Part model, mm, in its own coordinate system. A direction names the side the tool comes from. Give positions to 0.01 mm unless a question says otherwise; leave off trailing zeros. Write each loop counter-clockwise with the first axis right and the second up, starting at its lowest first coordinate (ties: lowest second). Pieces come first, ordered by that corner, then holes. Notation, with made-up numbers: M 8.5,-3.75 L 13.5,-3.75 A21 ccw 13.5,20.25 Z; hole C 28,-6.5 d11. An arc over 180 degrees is marked long. Answer as CSV lines item,"result". Start each with the question number.
1) Mould opens along X. For faces 1 (the flat face through (0, -17.5, -2)), 2 (the flat face through (-14.5, 0, -2)), 3 (the flat face through (17.5, 0, -2)) say: pulls with the +X half, pulls with the -X half, needs draft (parallel to the pull), parting line crosses it, or undercut.
2) Pin check, flat tip, straight feed: pin 1 Ø5 at (y, z) = (0, 56) entering from +X. Stop position of the tip, or through.
3) Slice it at A-A, the plane y = -12. Give the cut face in (x, z), plus the area to 3 significant figures.
4) Slice it at B-B, the plane z = 56. Give the cut face in (x, y), plus the area to 3 significant figures.
5) Slice it at D-D, the plane y = 0. Give the cut face in (x, z), plus the area to 3 significant figures.
6) Tool access for faces 4 (the flat face through (0, 14.5, -2)), 5 (the flat face through (-17.5, 0, -2)): list every direction of +Z, -Z, +X, -X, +Y, -Y with a clear straight run to the whole face (end or side of a thin tool).
7) Wall check: line 1 along Y through (x, z) = (15.8, 56); line 2 along X through (y, z) = (-11, -101.5). Give the ranges that are in metal, low to high. Write a range as from..to.
```python
from build123d import *

# Parameters (mm, degrees)
EXTRUDE_THIN1_DEPTH      = 140
EXTRUDE_THIN1_DEPTH_BACK = 140
SKETCH1_W                = 35
SKETCH1_H                = 35
SKETCH1_W_2              = 29
SKETCH1_H_2              = 29
FILLET1_R                = 2
SKETCH2_R                = 4
CUT_EXTRUDE1_DEPTH       = 40


with BuildPart() as part:
    # Sketch1 → Extrude-Thin1 (new, two sides: drawn at the far end of the back side and taken through both)
    with BuildSketch(Plane.XY.offset(-EXTRUDE_THIN1_DEPTH_BACK)):
        Rectangle(SKETCH1_W, SKETCH1_H)
        Rectangle(SKETCH1_W_2, SKETCH1_H_2, mode=Mode.SUBTRACT)
    extrude(amount=EXTRUDE_THIN1_DEPTH + EXTRUDE_THIN1_DEPTH_BACK)

    # Fillet1
    fillet1_edges = [part.edges().sort_by_distance(p)[0] for p in [
        (17.5, -17.5, 0),
        (-17.5, -17.5, 0),
        (-17.5, 17.5, 0),
        (17.5, 17.5, 0),
    ]]
    fillet(fillet1_edges, radius=FILLET1_R)

    # Sketch2 → Cut-Extrude1 (cut)
    with BuildSketch(Plane(origin=(17.5, 0, 0), x_dir=(0, 0, -1), z_dir=(1, 0, 0))):
        with Locations(Location((-56, 0, 0), (0, 0, 180))):
            Circle(SKETCH2_R)
    extrude(amount=-CUT_EXTRUDE1_DEPTH, mode=Mode.SUBTRACT)


solid = part.part
```
Found:
1,face 1,"needs draft"
1,face 2,"undercut"
1,face 3,"pulls with the +X half"
2,pin 1,"through"
3,outline,"M -17.5,-140 L -14.5,-140 L -14.5,140 L -17.5,140 Z; M 14.5,-140 L 17.5,-140 L 17.5,140 L 14.5,140 Z"
3,area,"1,680 mm²"
4,outline,"M -17.5,-15.5 A2 ccw -15.5,-17.5 L 15.5,-17.5 A2 ccw 17.5,-15.5 L 17.5,-4 L 14.5,-4 L 14.5,-14.5 L -14.5,-14.5 L -14.5,-4 L -17.5,-4 Z; M -17.5,4 L -14.5,4 L -14.5,14.5 L 14.5,14.5 L 14.5,4 L 17.5,4 L 17.5,15.5 A2 ccw 15.5,17.5 L -15.5,17.5 A2 ccw -17.5,15.5 Z"
4,area,"333 mm²"
5,outline,"M -17.5,-140 L -14.5,-140 L -14.5,52 L -17.5,52 Z; M -17.5,60 L -14.5,60 L -14.5,140 L -17.5,140 Z; M 14.5,-140 L 17.5,-140 L 17.5,52 L 14.5,52 Z; M 14.5,60 L 17.5,60 L 17.5,140 L 14.5,140 Z"
5,area,"1,630 mm²"
6,face 4,"+Z, -Z"
6,face 5,"+Z, -Z, -X, +Y, -Y"
7,line 1,"-17.48..-4, 4..17.48"
7,line 2,"-17.5..-14.5, 14.5..17.5"
